Model file for the job. Use its own axes, mm. Face numbers are marked on the shaded views. Round coordinates to 2 decimals unless told otherwise and drop trailing zeros. Write each loop counter-clockwise with the first axis right and the second up, starting at its lowest first coordinate (ties: lowest second). Pieces come first, ordered by that corner, then holes. Notation, with made-up numbers: (-15, 74.5) - (-9, 74.5) arc R7 ccw to (-9, 86.5) - close; hole circle Ø5 at (70.25, -32.75). An arc over 180 degrees is marked (long way). One line per item, written item: value.
from build123d import *


with BuildPart() as f1:
    # F0 (on Front) → F1 (revolve)
    with BuildSketch(Plane.XZ):
        Polygon((-5, 5), (-5, 0), (5, 0), (5, 5), (2.5, 5), (-2.5, 5), align=None)
        Polygon((-5, 12.5), (-5, 5), (-2.5, 5), (2.5, 5), (5, 5), (5, 12.5), (2.5, 12.5), (-2.5, 12.5), align=None)
        Polygon((-5, 17.5), (-5, 12.5), (-2.5, 12.5), (2.5, 12.5), (5, 12.5), (5, 17.5), (3.75, 17.5), (2.5, 15.500004), (-2.5, 15.500004), (-3.75, 17.5), align=None)
    revolve(axis=Axis((0.313021, 0, -2.5), (1, 0, 0)))


solid = f1.part
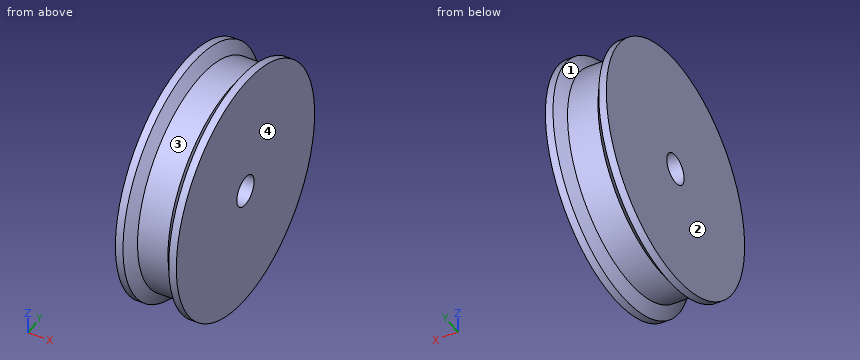
1. Mould opens along X. For the marked faces 1, 2, 3 and 4 say: released by +X, released by -X, zero draft, split by the parting line, or undercut.
Report:
face 1: undercut
face 2: released by -X
face 3: undercut
face 4: released by +X
2. Drop flat-ended pins along their axis: pin 1 (1 mm diameter, centred on x = 1.5, z = -16, fed in from +Y); pin 2 (1 mm diameter, centred on x = 1.5, z = 1.5, fed in from +Y); pin 3 (4 mm diameter, centred on x = 2, z = -11, fed in from +Y). Give the stop position or say it passes through.
Report:
pin 1: y = 12.45
pin 2: y = 17.66
pin 3: y = 18.53
3. Wall check: probe 1 along Y at (x, z) = (-0.5, -2.5); probe 2 along Z at (x, y) = (1, 0); probe 3 along X at (y, z) = (-11.5, -17.5). Give the ranges that are in metal, low to high. Write a range as [from, to].
Report:
probe 1: [-18, -2.5], [2.5, 18]
probe 2: [-20.5, -5], [0, 15.5]
probe 3: [-5, -3.06], [3.06, 5]
4. Band-saw the part on C-C on x = -1.5. Write the cut outline in (y, z), plus the area to 3 significant figures.
Report:
outline: circle Ø36 at (0, -2.5); hole circle Ø5 at (0, -2.5)
area: 998 mm²
5. Band-saw the part on B-B on y = 0. Write the cut outline in (x, z).
Report:
outline: (-5, -22.5) - (-3.75, -22.5) - (-2.5, -20.5) - (2.5, -20.5) - (3.75, -22.5) - (5, -22.5) - (5, -5) - (-5, -5) - close; (-5, 0) - (5, 0) - (5, 17.5) - (3.75, 17.5) - (2.5, 15.5) - (-2.5, 15.5) - (-3.75, 17.5) - (-5, 17.5) - close
6. Band-saw the part on A-A on z = -2.5. Write the cut outline in (x, y), plus the area to 3 significant figures.
Report:
outline: (-5, -20) - (-3.75, -20) - (-2.5, -18) - (2.5, -18) - (3.75, -20) - (5, -20) - (5, -2.5) - (-5, -2.5) - close; (-5, 2.5) - (5, 2.5) - (5, 20) - (3.75, 20) - (2.5, 18) - (-2.5, 18) - (-3.75, 20) - (-5, 20) - close
area: 325 mm²
